```python
from build123d import *

# Parameters (mm, degrees)
F0_W      = 90
F0_H      = 187
F1_DEPTH  = 52
F2_T      = -12
F3_W      = 50
F3_H      = 40
F4_DEPTH  = 25
F5_R      = 2.25
F5_R_2    = 2.75
F6_DEPTH  = 52.001
F7_R      = 5
F8_DEPTH  = 6
F9_R      = 4.25
F10_DEPTH = 4.5
F11_R     = 2.5
F12_DEPTH = 100
F13_W     = 82
F13_H     = 3.25
F14_DEPTH = 180


with BuildPart() as f1:
    # F0 (on Front) → F1 (new body)
    with BuildSketch(Plane.XZ):
        with Locations((45, 93.5)):
            Rectangle(F0_W, F0_H)
    extrude(amount=F1_DEPTH)

    # F2
    f2_openings = [f1.faces().sort_by_distance(p)[0] for p in [
        (45, -52, 93.5),
        (45, -26, 0),
    ]]
    offset(amount=F2_T, openings=f2_openings)

    # F3 (on face) → F4 (cut)
    with BuildSketch(Plane.XY.offset(187)):
        with Locations((45, -32)):
            Rectangle(F3_W, F3_H)
    extrude(amount=-F4_DEPTH, mode=Mode.SUBTRACT)

    # F5 (on face) → F6 (cut, through all)
    with BuildSketch(Plane(origin=(0, 0, 0), x_dir=(-1, 0, 0), z_dir=(0, 1, 0))):
        with Locations((-65, 53)):
            Circle(F5_R)
        with Locations((-25, 53)):
            Circle(F5_R)
        with Locations((-65, 153)):
            Circle(F5_R)
        with Locations((-25, 153)):
            Circle(F5_R)
        with Locations((-26, 120.5)):
            Circle(F5_R_2)
        with Locations((-64, 120.5)):
            Circle(F5_R_2)
        with Locations((-26, 90.5)):
            Circle(F5_R_2)
        with Locations((-64, 90.5)):
            Circle(F5_R_2)
    extrude(amount=-F6_DEPTH, mode=Mode.SUBTRACT)

    # F7 (on face) → F8 (cut)
    with BuildSketch(Plane.XZ.offset(12)):
        with Locations((26, 120.5)):
            Circle(F7_R)
        with Locations((64, 120.5)):
            Circle(F7_R)
        with Locations((26, 90.5)):
            Circle(F7_R)
        with Locations((64, 90.5)):
            Circle(F7_R)
    extrude(amount=-F8_DEPTH, mode=Mode.SUBTRACT)

    # F9 (on face) → F10 (cut)
    with BuildSketch(Plane(origin=(0, 0, 0), x_dir=(-1, 0, 0), z_dir=(0, 1, 0))):
        with Locations((-65, 153)):
            Circle(F9_R)
        with Locations((-25, 153)):
            Circle(F9_R)
        with Locations((-65, 53)):
            Circle(F9_R)
        with Locations((-25, 53)):
            Circle(F9_R)
    extrude(amount=-F10_DEPTH, mode=Mode.SUBTRACT)

    # F11 (on face) → F12 (cut)
    with BuildSketch(Plane(origin=(0, 0, 0), x_dir=(1, 0, 0), z_dir=(0, 0, -1))):
        with Locations((6, 25)):
            Circle(F11_R)
        with Locations((84, 25)):
            Circle(F11_R)
    extrude(amount=-F12_DEPTH, mode=Mode.SUBTRACT)

    # F13 (on face) → F14 (cut)
    with BuildSketch(Plane.XY.offset(187)):
        with Locations((45, -47.625)):
            Rectangle(F13_W, F13_H)
    extrude(amount=-F14_DEPTH, mode=Mode.SUBTRACT)


solid = f1.part
```
Read the model definition and answer for the solid it produces. Units are mm, in the model's axes. A direction names the side the tool comes from. Give positions to 0.01 mm unless a question says otherwise; leave off trailing zeros. Order: outer loops, then holes, each group sorted by start corner. A loop starts at its lowest first (then second) coordinate and runs counter-clockwise, first axis right, second up.
(1) For faces 5 (the flat face through (84, -25, 100)), 6 (the flat face through (78, -32, 86)), 7 (the cylindrical face through (63.04, -2.22, 49.23)), 8 (the flat face through (8, -49.25, 98)), 9 (the cylindrical face through (21.005, -9.042, 120.72)), determine the directions among +Z, -Z, +X, -X, +Y, -Y from which every point of the face is accessible in a straight line to the end or side of a thin tool.
(2) Find section C-C (z = 26.5). Give the vertices of the cut face in (x, y), plus the area to 3 significant figures.
(3) Straight lines are drawn through the part: L1, parallel to X at y = -47, z = 178; L2, parallel to Z at x = 65, y = -2; L3, parallel to Z at x = 25.5, y = -10.5. For each, find the intervals that lie inside material, in ascending order.
(4) For a pull along Y with two mould halves and no side action, classify faces 1 (the cylindrical face through (25.92, -2.22, 48.85)), 2 (the flat face through (86, -48, 98)), 3 (the flat face through (81, -46, 98)), 4 (the flat face through (23, -4.5, 51)) as released by +Y, released by -Y, zero draft, split by the parting line, or undercut.
(5) Find section A-A (z = 90.5). Give the number of separate pieces and of enclosed holes in the cut face, plus the area to 3 significant figures.
(6) Given pin 1 (2.5 mm diameter, centred on x = 26.5, z = 151, fed in from +Y); pin 2 (5 mm diameter, centred on x = 47, z = 60.5, fed in from -Y); pin 3 (1.6 mm diameter, centred on x = 82, y = -48, fed in from +Z), each flat-ended and moving along its own axis, determine where each tip first touches the part or whether it passes through.
(7) Find section B-B (y = -25). Give the vertices of the cut face in (x, z), plus the area to 3 significant figures.
Result sheet:
1. face 5: -Z
1. face 6: -Z, -Y
1. face 7: +Y
1. face 8: +Z
1. face 9: -Y
2. outline: (0, -52) - (12, -52) - (12, -49.25) - (4, -49.25) - (4, -46) - (12, -46) - (12, -12) - (78, -12) - (78, -46) - (86, -46) - (86, -49.25) - (78, -49.25) - (78, -52) - (90, -52) - (90, 0) - (0, 0) - close; hole circle Ø5 at (6, -25); hole circle Ø5 at (84, -25)
2. area: 1,950 mm2
3. L1: x = 0 to 4, 86 to 90
3. L2: z = 0 to 48.75, 57.25 to 87.94, 93.06 to 117.94, 123.06 to 148.75, 157.25 to 187
3. L3: z = 0 to 50.81, 55.19 to 85.53, 95.47 to 115.53, 125.47 to 150.81, 155.19 to 187
4. face 1: zero draft
4. face 2: undercut
4. face 3: undercut
4. face 4: released by +Y
5. separate pieces: 3
5. enclosed holes: 2
5. area: 1,760 mm2
6. pin 1: stops at y = -4.5
6. pin 2: stops at y = -12
6. pin 3: stops at z = 7
7. outline: (0, 0) - (3.5, 0) - (3.5, 100) - (8.5, 100) - (8.5, 0) - (12, 0) - (12, 175) - (20, 175) - (20, 187) - (0, 187) - close; (70, 175) - (78, 175) - (78, 0) - (81.5, 0) - (81.5, 100) - (86.5, 100) - (86.5, 0) - (90, 0) - (90, 187) - (70, 187) - close
7. area: 3,680 mm2
